Geometry check sheet. Reference: drawing and pictorial views, mm from the part's lowest x, y, z. A direction names the side the tool comes from. Round coordinates to 2 decimals unless told otherwise and drop trailing zeros. Loops run counter-clockwise (first coordinate to the right, second up) from the corner with the lowest first, then second, coordinate; pieces in that order, holes last. Notation, with made-up numbers: (52.5, 19) - (78.5, 19) arc R13 cw to (78.5, 33) - close; hole circle Ø2 at (-29.5, 65). An arc over 180 degrees is marked (long way). Put each result on its own line as item: value. Start each with the question number.
Item 1: Section check A-A, the plane x = 4.25. Record the cut outline in (y, z).
Item 2: Section check C-C, the plane z = 12.5. Record the cut outline in (x, y).
Item 3: Section check D-D, the plane y = 4.75. Record the cut outline in (x, z) (3 decimals), and give its area (3 significant figures).
Item 4: Section check B-B, the plane x = 9.5. Record the cut outline in (y, z), and give its area (3 significant figures).
Item 5: Tool access check on the marked faces 1 and 2. Record the directions out of +Z, -Z, +X, -X, +Y, -Y that give a thin tool (end or side, any length) a straight path to the whole face; none if there is none.
Item 6: Draft check along Z on the marked faces 3, 4 and 5. Enter one of: pulls with the +Z half, pulls with the -Z half, needs draft (parallel to the pull), parting line crosses it, or undercut.
Item 7: Material ranges on line 1 along Y through (x, z) = (3.5, 4.5); line 2 along X through (y, z) = (5.25, 8.75); line 3 along Z through (x, y) = (4.5, 5.5), recorded low to high.
Item 8: Gauge pin test, flat ends, axial feed: pin 1 Ø2 at (x, z) = (12, 9.5) entering from +Y; pin 2 Ø1.8 at (x, z) = (14.605, 9.525) entering from +Y; pin 3 Ø1.5 at (x, y) = (10, 0.5) entering from -Z (3 decimals). Record the tip position at first contact, or that the pin passes through.
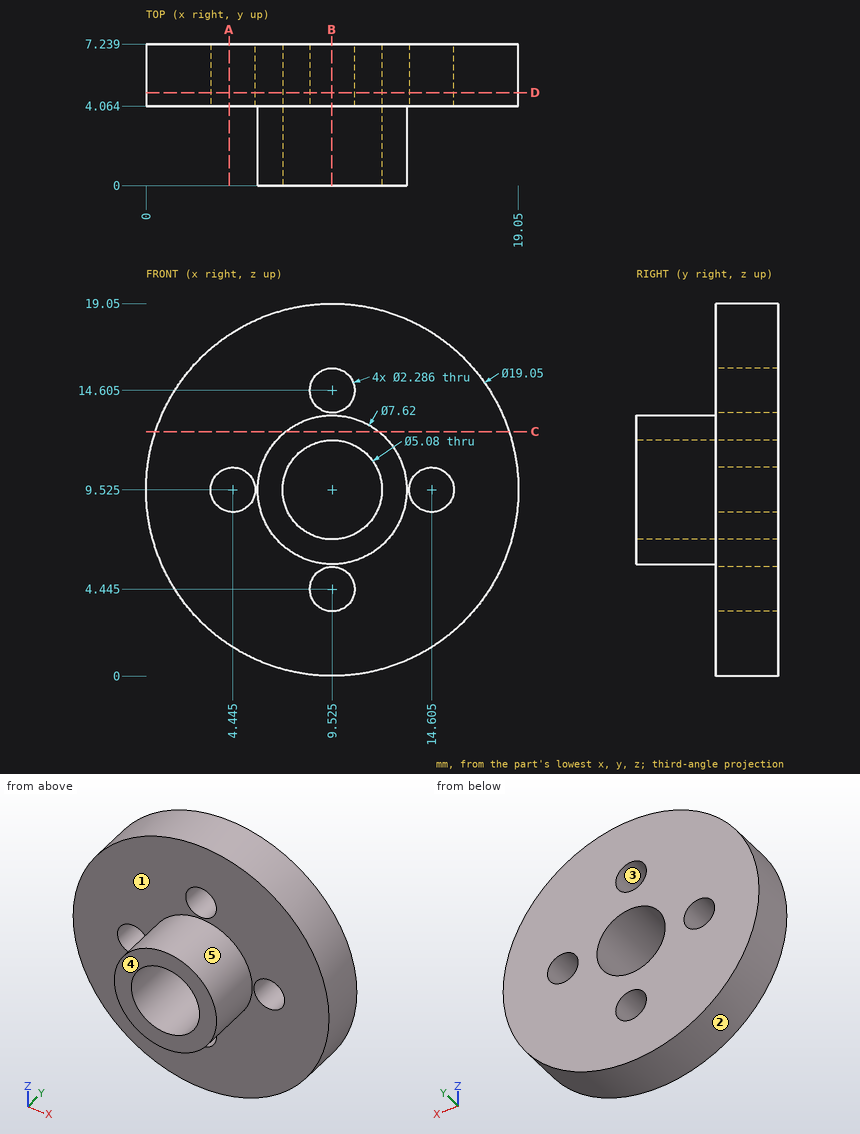
Check result:
1. outline: (4.06, 1.59) - (7.24, 1.59) - (7.24, 8.4) - (4.06, 8.4) - close; (4.06, 10.65) - (7.24, 10.65) - (7.24, 17.46) - (4.06, 17.46) - close
2. outline: (0.48, 4.06) - (7.14, 4.06) - (7.14, 0) - (11.91, 0) - (11.91, 4.06) - (18.57, 4.06) - (18.57, 7.24) - (0.48, 7.24) - close
3. outline: circle Ø19.05 at (9.525, 9.525); hole circle Ø2.286 at (4.445, 9.525); hole circle Ø5.08 at (9.525, 9.525); hole circle Ø2.286 at (9.525, 4.445); hole circle Ø2.286 at (9.525, 14.605); hole circle Ø2.286 at (14.605, 9.525)
3. area: 248 mm²
4. outline: (0, 5.72) - (4.06, 5.72) - (4.06, 5.59) - (7.24, 5.59) - (7.24, 6.99) - (0, 6.99) - close; (0, 12.06) - (7.24, 12.06) - (7.24, 13.46) - (4.06, 13.46) - (4.06, 13.33) - (0, 13.33) - close; (4.06, 0) - (7.24, 0) - (7.24, 3.3) - (4.06, 3.3) - close; (4.06, 15.75) - (7.24, 15.75) - (7.24, 19.05) - (4.06, 19.05) - close
4. area: 40.2 mm²
5. face 1: -Y
5. face 2: +Y, -Y
6. face 3: undercut
6. face 4: needs draft
6. face 5: parting line crosses it
7. line 1: 4.06 to 7.24
7. line 2: 0.03 to 3.6, 5.29 to 7.11, 11.94 to 13.76, 15.45 to 19.02
7. line 3: 1.43 to 8.38, 10.67 to 17.62
8. pin 1: y = 7.24
8. pin 2: through
8. pin 3: z = 5.715
